The drawing under review shows one solid part. Ordinate dimensions are in mm from its lowest x, y, z. Round coordinates to 2 decimals unless told otherwise and drop trailing zeros. Write each loop counter-clockwise with the first axis right and the second up, starting at its lowest first coordinate (ties: lowest second). Pieces come first, ordered by that corner, then holes. Notation, with made-up numbers: (-20, -28) -> (8, -28) arc R16 ccw to (8, -16) -> close; hole circle Ø6 at (75, 43). An arc over 180 degrees is marked (long way). Answer in a Markdown table with one row per item.
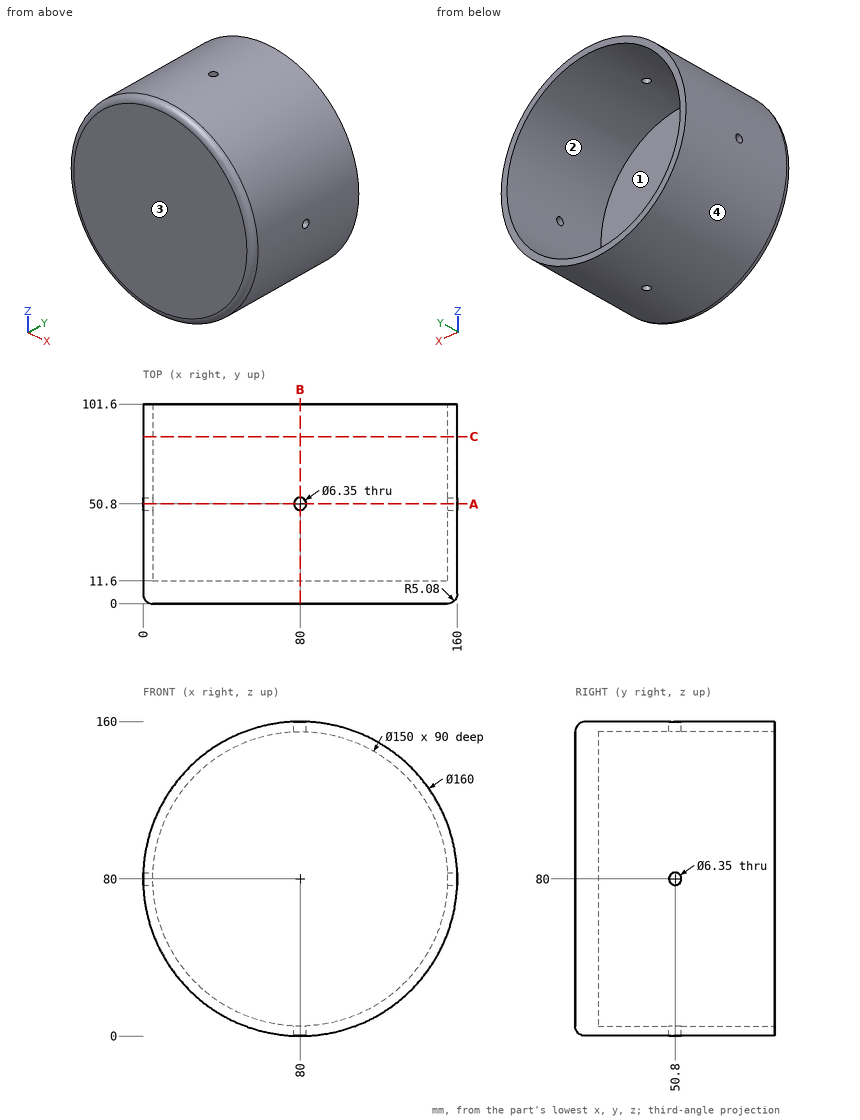
1) Consider section C-C on y = 85. State the section outline as (x, z) points, then the cut area to 3 significant figures.
Solved:
| item | result |
|---|---|
| outline | circle Ø160 at (80, 80); hole circle Ø150 at (80, 80) |
| area | 2,430 mm² |
2) Consider section A-A on y = 50.8. State the section outline as (x, z) points (3 decimals).
Solved:
| item | result |
|---|---|
| outline | (0.063, 76.825) arc R80 ccw to (76.825, 0.063) -> (76.825, 5.067) arc R75 cw to (5.067, 76.825) -> close; (0.063, 83.175) -> (5.067, 83.175) arc R75 cw to (76.825, 154.933) -> (76.825, 159.937) arc R80 ccw to start; (83.175, 0.063) arc R80 ccw to (159.937, 76.825) -> (154.933, 76.825) arc R75 cw to (83.175, 5.067) -> close; (83.175, 154.933) arc R75 cw to (154.933, 83.175) -> (159.937, 83.175) arc R80 ccw to (83.175, 159.937) -> close |
3) Mouldability with a two-part tool opening along Z and no side actions: class the marked faces 1, 2, 3 and 4 as pulls with the +Z half, pulls with the -Z half, needs draft (parallel to the pull), parting line crosses it, or undercut.
Solved:
| item | result |
|---|---|
| face 1 | undercut |
| face 2 | undercut |
| face 3 | needs draft |
| face 4 | parting line crosses it |
4) Clearance check with flat-ended pins moving along their axes: pin 1 Ø10 at (x, y) = (80, 50.8) entering from -Z; pin 2 Ø1.5 at (y, z) = (46.5, 124) entering from +X; pin 3 Ø5 at (x, y) = (22.5, 55) entering from -Z; pin 4 Ø8 at (y, z) = (32.5, 115) entering from -X. State where each tip first meets the part, or that it passes through.
Solved:
| item | result |
|---|---|
| pin 1 | z = 0 |
| pin 2 | x = 147.3 |
| pin 3 | z = 21.91 |
| pin 4 | x = 6.25 |
5) Consider section B-B on x = 80. State how many separate pieces and enclosed holes the cut face has, then the cut area to 3 significant figures.
Solved:
| item | result |
|---|---|
| separate pieces | 3 |
| enclosed holes | 0 |
| area | 2,680 mm² |
6) For line 1 (Z direction, x = 77.5, y = 80); line 2 (Y direction, x = 143, z = 98); line 3 (Z direction, x = 147.5, y = 59), list the stretches that pass through material, from the lowest coordinate up. Write a range as [from, to].
Solved:
| item | result |
|---|---|
| line 1 | [0.04, 5.04], [154.96, 159.96] |
| line 2 | [0, 11.6] |
| line 3 | [37.06, 47.31], [112.69, 122.94] |
